Autodesk Inventor part; units mm, degrees
ref_plane "YZ Plane" through (0, 0, 0) normal (1, 0, 0) x (0, 1, 0)
ref_plane "XZ Plane" through (0, 0, 0) normal (0, 1, 0) x (-1, 0, 0)
ref_plane "XY Plane" through (0, 0, 0) normal (0, 0, 1) x (1, 0, 0)
sketch "Boceto1" plane through (0, 0, 0) normal (0, 0, 1) x (1, 0, 0)
  circle A0 centre (0, 0) radius 1.5
  circle A1 centre (0, 0) radius 2.75
  dimension "d0" = 3
  dimension "d1" = 5.5
extrude "Extrusión1" add sketch "Boceto1" along normal blind 20 contours A0
extrude "Extrusión2" add sketch "Boceto1" against normal blind 2.5 contours A0 | A1
sketch "Boceto2" plane through (0, 0, -2.5) normal (0, 0, -1) x (-1, 0, 0)
  line L0 (1.5, 0) -> (0.75, -1.299)
  line L1 (0.75, -1.299) -> (-0.75, -1.299)
  line L2 (-0.75, -1.299) -> (-1.5, 0)
  line L3 (-1.5, 0) -> (-0.75, 1.299)
  line L4 (-0.75, 1.299) -> (0.75, 1.299)
  line L5 (0.75, 1.299) -> (1.5, 0)
  point P0 (0, 0)
  point P1 (0, 0)
  dimension "d6" = 3
fillet "Empalme1" radius 2 1 edges at (-2.75, 0, -2.5)
extrude "Extrusión4" cut sketch "Boceto2" against normal blind 1.5
thread "Rosca1"
properties part number "tonrilloM3x20mm" material "Acero inoxidable"
Could you check a few things on this model? Use its own coordinates, in mm. A direction names the side the tool comes from. Give positions to 0.01 mm unless a question says otherwise; leave off trailing zeros. Write each loop counter-clockwise with the first axis right and the second up, starting at its lowest first coordinate (ties: lowest second). Pieces come first, ordered by that corner, then holes. Notation, with made-up numbers: (44, -15.5) - (56, -15.5) arc R19 ccw to (56, 4.5) - close; hole circle Ø9 at (48.25, 62.25). An arc over 180 degrees is marked (long way). One line per item, written item: value. Start each with the question number.
Item 1: Imagine slicing it at A-A, the plane z = 7. List the corners of the cut face in (x, y) for me.
Item 2: I'm going to push flat-ended pins straight in: pin 1 (1.5 mm diameter, centred on x = -0.5, y = 0, fed in from -Z); pin 2 (0.7 mm diameter, centred on x = 0.5, z = -2, fed in from -Y); pin 3 (0.7 mm diameter, centred on x = 0, z = -1.5, fed in from +Y). Where does each tip first touch, or does it pass through?
Item 3: Which directions (+Z, -Z, +X, -X, +Y, -Y) give clear straight access to the entire face, cutting with the end or side of a thin tool? Please do faces 1 (the face through (-1.12, 0.66, -1.72)), 2 (the face through (-0.596, -2.685, -0.246)), 3 (the face through (1.2, -1.2, 0)).
Item 4: Please list where these lines run through material, in increasing order: line 1 (Z direction, x = -1.4, y = -2.05); line 2 (Z direction, x = 1.2, y = 0.35); line 3 (X direction, y = -0.75, z = 0.75). Write a range as from..to.
Geometry says:
1. outline: circle Ø3 at (0, 0)
2. pin 1: z = -1
2. pin 2: y = -2.34
2. pin 3: y = 2.64
3. face 1: -Z
3. face 2: +Z, -Z
3. face 3: +Z
4. line 1: -1.5..0
4. line 2: -1..20
4. line 3: -1.3..1.3
